```python
from build123d import *

# Parameters (mm, degrees)
SKETCH1_R           = 12.7
SKETCH1_R_2         = 10.668
BOSS_EXTRUDE1_DEPTH = 76.2
SKETCH2_R           = 12.7
SKETCH2_R_2         = 10.668
BOSS_EXTRUDE2_DEPTH = 38.1


with BuildPart() as part:
    # Sketch1 → Boss-Extrude1 (new body)
    with BuildSketch(Plane.XY):
        Circle(SKETCH1_R)
        Circle(SKETCH1_R_2, mode=Mode.SUBTRACT)
    extrude(amount=BOSS_EXTRUDE1_DEPTH)

    # Sketch2 → Boss-Extrude2 (add, symmetric)
    with BuildSketch(Plane(origin=(0, 0, 0), x_dir=(0, 0, -1), z_dir=(1, 0, 0))):
        with Locations((-42.5958, 0)):
            Circle(SKETCH2_R)
        with Locations((-42.5958, 0)):
            Circle(SKETCH2_R_2, mode=Mode.SUBTRACT)
    extrude(amount=BOSS_EXTRUDE2_DEPTH, both=True)


solid = part.part
```
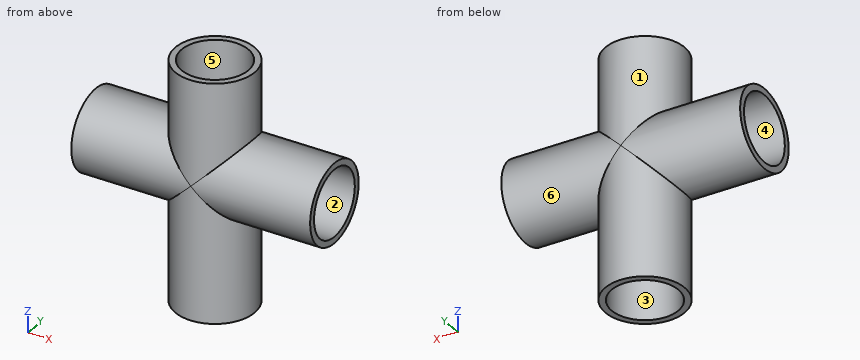
Here's how the part is built. I have some questions about the finished solid (model axes, mm). Face numbers are marked on the shaded views. A direction names the side the tool comes from. Round coordinates to 2 decimals unless told otherwise and drop trailing zeros. Loops run counter-clockwise (first coordinate to the right, second up) from the corner with the lowest first, then second, coordinate; pieces in that order, holes last.
1. Suppose I cut it at C-C, the plane z = 62. Please give me the cut outline in (x, y), and give its area (3 significant figures).
Answers:
outline: circle Ø25.4 at (0, 0); hole circle Ø21.34 at (0, 0)
area: 149 mm2
2. If I drill on probe 1 along Z at (x, y) = (15.5, -0.5); probe 2 along Y at (x, z) = (0, 62), over which ranges is the centre line in solid material (lowest first)?
Answers:
probe 1: z = 29.91 to 31.94, 53.25 to 55.29
probe 2: y = -12.7 to -10.67, 10.67 to 12.7
3. Thinking about a two-plate mould opening in Y: for the marked faces 5 and 6, which applies, released by +Y, released by -Y, zero draft, split by the parting line, or undercut?
Answers:
face 5: undercut
face 6: split by the parting line
4. Will these pins go through, and if not, where does the flat tip stop? pin 1 (10 mm diameter, centred on y = 3, z = 26, fed in from +X); pin 2 (3 mm diameter, centred on y = -4.5, z = 26.5, fed in from -X); pin 3 (8 mm diameter, centred on y = -7.5, z = 13, fed in from +X); pin 4 (2 mm diameter, centred on y = 1, z = 19, fed in from -X).
Answers:
pin 1: stops at x = 38.1
pin 2: stops at x = -12.34
pin 3: stops at x = 12.21
pin 4: stops at x = -12.7
5. For the marked faces 1, 2, 3 and 4, which set-ups out of +Z, -Z, +X, -X, +Y, -Y let a thin tool reach every point of the face, with its end or its side?
Answers:
face 1: +Z
face 2: +X
face 3: -Z
face 4: -X
6. Suppose I cut it at B-B, the plane x = -4.5. Please give me the cut outline in (y, z), and give its area (3 significant figures).
Answers:
outline: (-11.88, 0) - (-9.67, 0) - (-9.67, 34.37) arc R12.7 ccw to (9.67, 34.37) - (9.67, 0) - (11.88, 0) - (11.88, 38.1) arc R12.7 ccw to (11.88, 47.1) - (11.88, 76.2) - (9.67, 76.2) - (9.67, 50.83) arc R12.7 ccw to (-9.67, 50.83) - (-9.67, 76.2) - (-11.88, 76.2) - (-11.88, 47.1) arc R12.7 ccw to (-11.88, 38.1) - close; hole (-9.67, 38.1) arc R10.67 ccw to (9.67, 38.1) - (9.67, 47.1) arc R10.67 ccw to (-9.67, 47.1) - close
area: 439 mm2
